Verification items for the finished model (mm, model axes). A direction names the side the tool comes from. Round coordinates to 2 decimals unless told otherwise and drop trailing zeros. Write each loop counter-clockwise with the first axis right and the second up, starting at its lowest first coordinate (ties: lowest second). Pieces come first, ordered by that corner, then holes. Notation, with made-up numbers: (34.5, 38) - (67.5, 38) arc R25 cw to (67.5, 65) - close; hole circle Ø8 at (3, 78). An arc over 180 degrees is marked (long way). Write each question's results on one line, items separated by ' | '.
```python
from build123d import *

# Parameters (mm, degrees)
SKETCH1_W           = 40
SKETCH1_H           = 40
BOSS_EXTRUDE1_DEPTH = 4
SKETCH2_R           = 6.3
SKETCH2_R_2         = 1.5
CUT_EXTRUDE2_DEPTH  = 5
SKETCH3_R           = 18.5
CUT_EXTRUDE3_DEPTH  = 2


with BuildPart() as part:
    # Sketch1 → Boss-Extrude1 (new body)
    with BuildSketch(Plane(origin=(0, 0, 0), x_dir=(1, 0, 0), z_dir=(0, 1, 0))):
        Rectangle(SKETCH1_W, SKETCH1_H)
    extrude(amount=BOSS_EXTRUDE1_DEPTH)

    # Sketch2 → Cut-Extrude2 (cut)
    with BuildSketch(Plane(origin=(0, 4, 0), x_dir=(1, 0, 0), z_dir=(0, 1, 0))):
        with Locations(Location((0, -7, 0), (0, 0, 270))):
            Circle(SKETCH2_R)
        with Locations(Location((15.5, 0, 0), (0, 0, 270))):
            Circle(SKETCH2_R_2)
        with Locations(Location((7.75, -13.423393759, 0), (0, 0, 270))):
            Circle(SKETCH2_R_2)
        with Locations(Location((-7.75, -13.423393759, 0), (0, 0, 270))):
            Circle(SKETCH2_R_2)
        with Locations(Location((-15.5, 0, 0), (0, 0, 270))):
            Circle(SKETCH2_R_2)
        with Locations(Location((-7.75, 13.423393759, 0), (0, 0, 270))):
            Circle(SKETCH2_R_2)
        with Locations(Location((7.75, 13.423393759, 0), (0, 0, 270))):
            Circle(SKETCH2_R_2)
    extrude(amount=-CUT_EXTRUDE2_DEPTH, mode=Mode.SUBTRACT)

    # Sketch3 → Cut-Extrude3 (cut)
    with BuildSketch(Plane(origin=(0, 4, 0), x_dir=(1, 0, 0), z_dir=(0, 1, 0))):
        with Locations(Location((0, 0, 0), (0, 0, 270))):
            Circle(SKETCH3_R)
    extrude(amount=-CUT_EXTRUDE3_DEPTH, mode=Mode.SUBTRACT)


solid = part.part
```
(1) Section check A-A (y = 1.45). Record the cut outline in (x, z).
Answer:
outline: (-20, -20) - (20, -20) - (20, 20) - (-20, 20) - close; hole circle Ø3 at (-15.5, 0); hole circle Ø3 at (-7.75, -13.42); hole circle Ø3 at (-7.75, 13.42); hole circle Ø12.6 at (0, 7); hole circle Ø3 at (7.75, -13.42); hole circle Ø3 at (7.75, 13.42); hole circle Ø3 at (15.5, 0)
(2) Section check D-D (z = 7). Record the cut outline in (x, y).
Answer:
outline: (-20, 0) - (-6.3, 0) - (-6.3, 2) - (-17.12, 2) - (-17.12, 4) - (-20, 4) - close; (6.3, 0) - (20, 0) - (20, 4) - (17.12, 4) - (17.12, 2) - (6.3, 2) - close
(3) Set-up check for faces 1 (the cylindrical face through (-7.086, 3.014, 17.089)), 2 (the flat face through (-20, 2, 0)): record each of +Z, -Z, +X, -X, +Y, -Y from which the full face is reachable in a straight line by a thin tool's end or side.
Answer:
face 1: +Y | face 2: +Z, -Z, -X, +Y, -Y
(4) Go/stop test with flat-tipped pins: pin 1 Ø5 at (x, z) = (-7.75, 13.42) entering from +Y; pin 2 Ø7.5 at (x, z) = (0, 7) entering from +Y. Record where each tip stops, or that it passes through.
Answer:
pin 1: y = 2 | pin 2: through
(5) Mould release check, pull along X, two halves, no side actions. Record for faces 3 (the flat face through (20, 2, 0)), 4 (the cylindrical face through (0.277, 1.014, 0.706)), 5 (the flat face through (0, 0, 0)), 6 (the cylindrical face through (16.765, 1.014, 0.806)): released by +X, released by -X, zero draft, split by the parting line, or undercut.
Answer:
face 3: released by +X | face 4: undercut | face 5: zero draft | face 6: undercut
(6) Section check C-C (x = 3). Record the cut outline in (y, z).
Answer:
outline: (0, -20) - (4, -20) - (4, -18.26) - (2, -18.26) - (2, 1.46) - (0, 1.46) - close; (0, 12.54) - (2, 12.54) - (2, 18.26) - (4, 18.26) - (4, 20) - (0, 20) - close
(7) Section check B-B (z = 0). Record the cut outline in (x, y), plus the area to 3 significant figures.
Answer:
outline: (-20, 0) - (-17, 0) - (-17, 2) - (-18.5, 2) - (-18.5, 4) - (-20, 4) - close; (-14, 0) - (14, 0) - (14, 2) - (-14, 2) - close; (17, 0) - (20, 0) - (20, 4) - (18.5, 4) - (18.5, 2) - (17, 2) - close | area: 74.0 mm2
(8) Thickness scan on L1, parallel to X at y = 0.8, z = 0; L2, parallel to X at y = 2.75, z = 0; L3, parallel to X at y = 0.5, z = 7. Record the ranges inside material, lowest first.
Answer:
L1: -20 to -17, -14 to 14, 17 to 20 | L2: -20 to -18.5, 18.5 to 20 | L3: -20 to -6.3, 6.3 to 20
